```python
from build123d import *

# Parameters (mm, degrees)
SKETCH2_R           = 4
SKETCH2_R_2         = 11
BOSS_EXTRUDE1_DEPTH = 20
SKETCH3_R           = 7.5
CUT_EXTRUDE1_DEPTH  = 5
SKETCH4_R           = 20
SKETCH4_R_2         = 16
BOSS_EXTRUDE2_DEPTH = 10
CUT_EXTRUDE2_START  = -10
CUT_EXTRUDE2_DEPTH  = 10


with BuildPart() as part:
    # Sketch2 → Boss-Extrude1 (new body)
    with BuildSketch(Plane.XY):
        with BuildLine():
            Line((44.537767857, 44.08379372), (0, 30))
            ThreePointArc((0, 30), (-24.270509831, -17.633557569), (28.531695489, -9.270509831))
            Line((28.531695489, -9.270509831), (55.68910644, 28.735292906))
            ThreePointArc((55.68910644, 28.735292906), (55.642995759, 40.427002804), (44.537767857, 44.08379372))
        make_face()
        with Locations((47.552825815, 34.549150281)):
            Circle(SKETCH2_R, mode=Mode.SUBTRACT)
        Circle(SKETCH2_R_2, mode=Mode.SUBTRACT)
    extrude(amount=BOSS_EXTRUDE1_DEPTH)

    # Sketch3 → Cut-Extrude1 (cut)
    with BuildSketch(Plane(origin=(0, 0, 0), x_dir=(-1, 0, 0), z_dir=(0, 0, -1))):
        with Locations((-47.552825815, 34.549150281)):
            Circle(SKETCH3_R)
    extrude(amount=-CUT_EXTRUDE1_DEPTH, mode=Mode.SUBTRACT)

    # Sketch4 → Boss-Extrude2 (add)
    with BuildSketch(Plane(origin=(0, 0, 0), x_dir=(-1, 0, 0), z_dir=(0, 0, -1))):
        with Locations(Location((0, 0, 0), (0, 0, 180))):
            Circle(SKETCH4_R)
        Circle(SKETCH4_R_2, mode=Mode.SUBTRACT)
    extrude(amount=BOSS_EXTRUDE2_DEPTH)

    # Sketch5 → Cut-Extrude2 (cut)
    with BuildSketch(Plane.XY.offset(20).offset(CUT_EXTRUDE2_START)):
        with BuildLine():
            Line((44.537767857, 44.08379372), (0, 30))
            ThreePointArc((0, 30), (11.251062951, 8.174375719), (28.531695489, -9.270509831))
            Line((28.531695489, -9.270509831), (55.68910644, 28.735292906))
            ThreePointArc((55.68910644, 28.735292906), (55.642995759, 40.427002804), (44.537767857, 44.08379372))
        make_face()
    extrude(amount=CUT_EXTRUDE2_DEPTH, mode=Mode.SUBTRACT)


solid = part.part
```
For this review, take the finished solid that the model builds, in its own axes (mm). A direction names the side the tool comes from. Give positions to 0.01 mm unless a question says otherwise; leave off trailing zeros. Write each loop counter-clockwise with the first axis right and the second up, starting at its lowest first coordinate (ties: lowest second). Pieces come first, ordered by that corner, then holes. Notation, with made-up numbers: M 66,87 L 98,87 A10 ccw 98,91 Z; hole C 59,-36.75 d5. An arc over 180 degrees is marked long. Answer as a JSON object with one key per item and string values. Group by question number.
Item 1: Tool access review of faces 1 (the flat face through (28, 24, 10)), 2 (the flat face through (41.92, 9.466, 4.93)), 3 (the flat face through (3, 11, 0)): name each direction out of +Z, -Z, +X, -X, +Y, -Y from which nothing blocks a thin tool from reaching the whole face with its end or side.
Item 2: For probe 1 along X at (y, z) = (6, 2); probe 2 along Z at (x, y) = (51.5, 28.5); probe 3 along Y at (x, z) = (2, 12), list the stretches that pass through material, from the lowest coordinate up. Write a range as [from, to].
Item 3: Draft analysis for pull direction Y (two halves, no side actions). For faces 4 (the flat face through (-8, -13, 20)), 5 (the flat face through (22.58, 37.14, 4.93)), 6 (the cylindrical face through (3.47, -15.62, -4.93)), state which applies: +Y half, -Y half, draft (parallel to the pull), parting line (faces both ways), or undercut.
Item 4: Consider section A-A on y = -2. Write out the cut boundary in (x, z).
Item 5: Consider section D-D on x = 26. Write out the cut boundary in (y, z).
Item 6: Consider section C-C on z = -7. Write out the cut boundary in (x, y), plus the area to 3 significant figures.
Item 7: Consider section B-B on x = -1. Write out the cut boundary in (y, z), plus the area to 3 significant figures.
Item 8: For pin 1 Ø3 at (x, y) = (25.5, 6.5) entering from -Z; pin 2 Ø20 at (x, y) = (0, 0) entering from +Z; pin 3 Ø9 at (x, y) = (47.55, 34.55) entering from -Z; pin 4 Ø2 at (y, z) = (-15.5, 8) entering from -X, all flat-tipped, find the tip position at first contact; note any pin that passes through.
Check result:
{
 "1": {"face 1": "+Z, +X, +Y", "face 2": "+Z, -Z, +X, -Y", "face 3": "-Z"},
 "2": {"probe 1": "x = [-29.39, -9.22], [9.22, 39.44]", "probe 2": "z = [5, 10]", "probe 3": "y = [-29.93, -10.82], [10.82, 24.67]"},
 "3": {"face 4": "draft", "face 5": "+Y half", "face 6": "undercut"},
 "4": {"outline": "M -29.93,0 L -19.9,0 L -19.9,-10 L -15.87,-10 L -15.87,0 L -10.82,0 L -10.82,20 L -29.93,20 Z; M 10.82,0 L 15.87,0 L 15.87,-10 L 19.9,-10 L 19.9,0 L 33.73,0 L 33.73,10 L 20.02,10 L 20.02,20 L 10.82,20 Z"},
 "5": {"outline": "M -14.97,0 L 38.22,0 L 38.22,10 L -7.32,10 L -7.32,20 L -14.97,20 Z"},
 "6": {"outline": "C 0,0 d40; hole C 0,0 d32", "area": "452 mm^2"},
 "7": {"outline": "M -29.98,0 L -19.97,0 L -19.97,-10 L -15.97,-10 L -15.97,0 L -10.95,0 L -10.95,20 L -29.98,20 Z; M 10.95,0 L 15.97,0 L 15.97,-10 L 19.97,-10 L 19.97,0 L 29.98,0 L 29.98,20 L 10.95,20 Z", "area": "841 mm^2"},
 "8": {"pin 1": "stops at z = 0", "pin 2": "passes through", "pin 3": "stops at z = 5", "pin 4": "stops at x = -26.26"}
}
